The listing builds one solid part. Answer for the finished solid, in the listing's coordinates (mm). Coordinates: 2 decimals unless noted, no trailing zeros. Order: outer loops, then holes, each group sorted by start corner. A loop starts at its lowest first (then second) coordinate and runs counter-clockwise, first axis right, second up. Notation, with made-up numbers: (-33.5, 59.25) -> (5.5, 59.25) arc R15 cw to (5.5, 65.25) -> close; hole circle Ø5 at (-34, -3). An arc over 180 degrees is marked (long way). Answer in a Markdown table with one row per item.
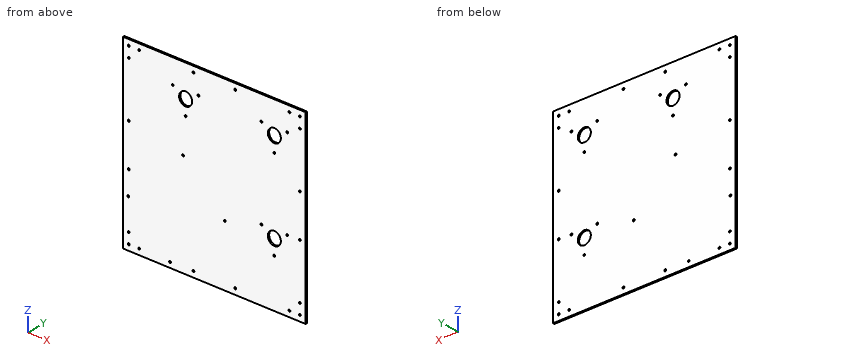
```python
from build123d import *

# Parameters (mm, degrees)
SKETCH_1_W               = 350
SKETCH_1_H               = 350
EXTRUDE_302_DEPTH        = 3
CUT_EXTRUDE_1_DEPTH      = 248.505555493
CUT_EXTRUDE_1_DEPTH_BACK = 248.505555493
SKETCH_2_R               = 1.75
SKETCH_2_R_2             = 12.5
SKETCH_3_R               = 1.75
PVC_DEPTH                = 248.505555493


with BuildPart() as part:
    # 草图1 → Extrude 302 (new body)
    with BuildSketch(Plane(origin=(0, 0, 0), x_dir=(1, 0, 0), z_dir=(0, 1, 0))):
        Rectangle(SKETCH_1_W, SKETCH_1_H)
    extrude(amount=EXTRUDE_302_DEPTH)

    # 草图2 → 切除-拉伸1 (cut, two sides: drawn at the far end of the back side and taken through both)
    with BuildSketch(Plane(origin=(0, 3, 0), x_dir=(1, 0, 0), z_dir=(0, 1, 0)).offset(-CUT_EXTRUDE_1_DEPTH_BACK)):
        with Locations(Location((20.060966544, 59.939033456, 0), (0, 0, 270))):
            Circle(SKETCH_2_R)
        with Locations(Location((-59.939033456, -20.060966544, 0), (0, 0, 270))):
            Circle(SKETCH_2_R)
        with Locations(Location((-165, 85, 0), (0, 0, 270))):
            Circle(SKETCH_2_R)
        with Locations(Location((-85, 165, 0), (0, 0, 270))):
            Circle(SKETCH_2_R)
        with Locations(Location((-55, -115, 0), (0, 0, 270))):
            Circle(SKETCH_2_R_2)
        with Locations(Location((115, -115, 0), (0, 0, 270))):
            Circle(SKETCH_2_R_2)
        with Locations(Location((115, 55, 0), (0, 0, 270))):
            Circle(SKETCH_2_R_2)
        with Locations(Location((-55, -86.5, 0), (0, 0, 270))):
            Circle(SKETCH_2_R)
        with Locations(Location((115, -86.5, 0), (0, 0, 270))):
            Circle(SKETCH_2_R)
        with Locations(Location((115, 83.5, 0), (0, 0, 270))):
            Circle(SKETCH_2_R)
        with Locations(Location((139.681724008, 40.75, 0), (0, 0, 270))):
            Circle(SKETCH_2_R)
        with Locations(Location((90.318275992, 40.75, 0), (0, 0, 270))):
            Circle(SKETCH_2_R)
        with Locations(Location((-30.318275992, -129.25, 0), (0, 0, 270))):
            Circle(SKETCH_2_R)
        with Locations(Location((-79.681724008, -129.25, 0), (0, 0, 270))):
            Circle(SKETCH_2_R)
        with Locations(Location((139.681724008, -129.25, 0), (0, 0, 270))):
            Circle(SKETCH_2_R)
        with Locations(Location((90.318275992, -129.25, 0), (0, 0, 270))):
            Circle(SKETCH_2_R)
    extrude(amount=CUT_EXTRUDE_1_DEPTH + CUT_EXTRUDE_1_DEPTH_BACK, mode=Mode.SUBTRACT)

    # 草图3 → PVC安装 (cut, through all)
    with BuildSketch(Plane(origin=(0, 3, 0), x_dir=(1, 0, 0), z_dir=(0, 1, 0))):
        with Locations(Location((-164, 144, 0), (0, 0, 270))):
            Circle(SKETCH_3_R)
        with Locations(Location((-164, 164, 0), (0, 0, 270))):
            Circle(SKETCH_3_R)
        with Locations(Location((-144, 164, 0), (0, 0, 270))):
            Circle(SKETCH_3_R)
        with Locations(Location((164, 164, 0), (0, 0, 270))):
            Circle(SKETCH_3_R)
        with Locations(Location((144, 164, 0), (0, 0, 270))):
            Circle(SKETCH_3_R)
        with Locations(Location((164, 144, 0), (0, 0, 270))):
            Circle(SKETCH_3_R)
        with Locations(Location((164, -164, 0), (0, 0, 270))):
            Circle(SKETCH_3_R)
        with Locations(Location((164, -144, 0), (0, 0, 270))):
            Circle(SKETCH_3_R)
        with Locations(Location((144, -164, 0), (0, 0, 270))):
            Circle(SKETCH_3_R)
        with Locations(Location((-164, -164, 0), (0, 0, 270))):
            Circle(SKETCH_3_R)
        with Locations(Location((-144, -164, 0), (0, 0, 270))):
            Circle(SKETCH_3_R)
        with Locations(Location((-164, -144, 0), (0, 0, 270))):
            Circle(SKETCH_3_R)
        with Locations(Location((-164, 40, 0), (0, 0, 270))):
            Circle(SKETCH_3_R)
        with Locations(Location((-164, -40, 0), (0, 0, 270))):
            Circle(SKETCH_3_R)
        with Locations(Location((40, 164, 0), (0, 0, 270))):
            Circle(SKETCH_3_R)
        with Locations(Location((-40, 164, 0), (0, 0, 270))):
            Circle(SKETCH_3_R)
        with Locations(Location((164, -40, 0), (0, 0, 270))):
            Circle(SKETCH_3_R)
        with Locations(Location((164, 40, 0), (0, 0, 270))):
            Circle(SKETCH_3_R)
        with Locations(Location((-40, -164, 0), (0, 0, 270))):
            Circle(SKETCH_3_R)
        with Locations(Location((40, -164, 0), (0, 0, 270))):
            Circle(SKETCH_3_R)
    extrude(amount=-PVC_DEPTH, mode=Mode.SUBTRACT)


solid = part.part
```
(1) Find the intervals of material crossed by line 1 along Z through (x, y) = (-144, 0.95); line 2 along X through (y, z) = (1.85, 129.25), in increasing order. Write a range as from..to.
Check values:
| item | result |
|---|---|
| line 1 | -175..-165.75, -162.25..162.25, 165.75..175 |
| line 2 | -175..-81.43, -77.93..-32.07, -28.57..88.57, 92.07..137.93, 141.43..175 |
(2) A cutting plane is placed at A-A, the plane x = 107.5. Determine the outline of the cut face in (y, z).
Check values:
| item | result |
|---|---|
| outline | (0, -175) -> (3, -175) -> (3, -65) -> (0, -65) -> close; (0, -45) -> (3, -45) -> (3, 105) -> (0, 105) -> close; (0, 125) -> (3, 125) -> (3, 175) -> (0, 175) -> close |
(3) A flat-ended cylindrical pin translates along its axis: pin 1 (4 mm diameter, centred on x = -65.5, z = -1.5, fed in from -Y). Find the tip coordinate at first contact, or state that the pin passes through.
Check values:
| item | result |
|---|---|
| pin 1 | y = 0 |
